from build123d import *

# Parameters (mm, degrees)
ESBO_O1_W                = 250
ESBO_O1_H                = 475
RESSALTO_EXTRUS_O1_DEPTH = 6
ESBO_O2_W                = 250
ESBO_O2_H                = 6
RESSALTO_EXTRUS_O2_DEPTH = 25
ESBO_O3_W                = 250
ESBO_O3_H                = 6
RESSALTO_EXTRUS_O4_DEPTH = 80
ESBO_O4_W                = 250
ESBO_O4_H                = 6
CORTE_EXTRUS_O1_DEPTH    = 70
ESBO_O5_R                = 3.3
ESBO_O5_R_2              = 9.2
ESBO_O5_R_3              = 5.5
CORTE_EXTRUS_O3_DEPTH    = 537.806296535


with BuildPart() as part:
    # Esboço1 → Ressalto-extrusão1 (new body)
    with BuildSketch(Plane(origin=(0, 0, 0), x_dir=(1, 0, 0), z_dir=(0, 1, 0))):
        with Locations((125, -237.5)):
            Rectangle(ESBO_O1_W, ESBO_O1_H)
    extrude(amount=RESSALTO_EXTRUS_O1_DEPTH)

    # Esboço2 → Ressalto-extrusão2 (add)
    with BuildSketch(Plane(origin=(0, 0, 0), x_dir=(-1, 0, 0), z_dir=(0, 0, -1))):
        with Locations((-125, 3)):
            Rectangle(ESBO_O2_W, ESBO_O2_H)
    extrude(amount=RESSALTO_EXTRUS_O2_DEPTH)

    # Esboço3 → Ressalto-extrusão4 (add)
    with BuildSketch(Plane(origin=(0, 0, -25), x_dir=(-1, 0, 0), z_dir=(0, 0, -1))):
        with Locations((-125, 3)):
            Rectangle(ESBO_O3_W, ESBO_O3_H)
    extrude(amount=RESSALTO_EXTRUS_O4_DEPTH)

    # Esboço4 → Corte-extrusão1 (cut)
    with BuildSketch(Plane(origin=(0, 0, -105), x_dir=(-1, 0, 0), z_dir=(0, 0, -1))):
        with Locations((-125, 3)):
            Rectangle(ESBO_O4_W, ESBO_O4_H)
    extrude(amount=-CORTE_EXTRUS_O1_DEPTH, mode=Mode.SUBTRACT)

    # Esboço5 → Corte-extrusão3 (cut, through all)
    with BuildSketch(Plane(origin=(0, 6, 0), x_dir=(1, 0, 0), z_dir=(0, 1, 0))):
        with Locations(Location((125, -142.97362902, 0), (0, 0, 270))):
            Circle(ESBO_O5_R)
        with Locations(Location((123.645994784, -156.588756812, 0), (0, 0, 270))):
            Circle(ESBO_O5_R_2)
        with Locations(Location((123.645994784, -192.796164786, 0), (0, 0, 270))):
            Circle(ESBO_O5_R_3)
        with Locations(Location((123.645994784, -176.121700588, 0), (0, 0, 270))):
            Circle(ESBO_O5_R_2)
    extrude(amount=-CORTE_EXTRUS_O3_DEPTH, mode=Mode.SUBTRACT)


solid = part.part
Input: part model. Units: mm. Frame: model coordinates. Round coordinates to 2 decimals unless told otherwise and drop trailing zeros. Answer as a JSON object with one key per item and string values. Group by question number.
1) Ray query, L1, parallel to Z at x = 132, y = 0.5; L2, parallel to Z at x = 131, y = 1.4. Return the intervals inside material, ascending.
2) Pin query (flat end, axial travel): pin 1 (5 mm diameter, centred on x = 97.5, z = 172, fed in from -Y); pin 2 (14.5 mm diameter, centred on x = 123.65, z = 176.12, fed in from -Y). Return the tip coordinate at first contact, or that it passes through.
3) Draft query along Z for faces 1 (the cylindrical face through (129.864, 3.042, 149.808)), 2 (the flat face through (127, 0, 224)). Return one class per face: +Z half, -Z half, draft (parallel to the pull), parting line (faces both ways), or undercut.
Reply:
{
 "1": {"L1": "z = -35 to 152.74, 160.44 to 172.27, 179.98 to 475", "L2": "z = -35 to 151.06, 162.12 to 170.59, 181.65 to 475"},
 "2": {"pin 1": "stops at y = 0", "pin 2": "passes through"},
 "3": {"face 1": "undercut", "face 2": "draft"}
}
